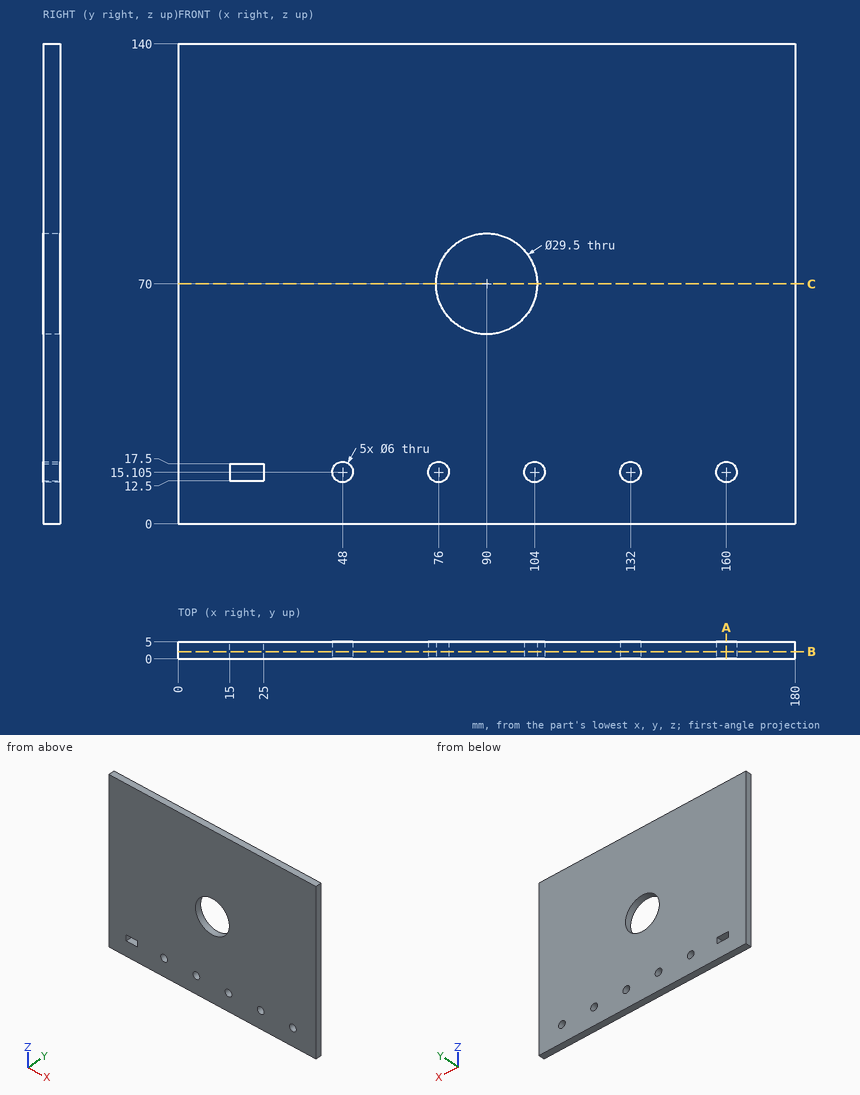
Study the drawing (mm; zero at the part's minimum x, y, z) and answer. Give positions to 0.01 mm unless a question says otherwise; leave off trailing zeros. Write each loop counter-clockwise with the first axis right and the second up, starting at its lowest first coordinate (ties: lowest second). Pieces come first, ordered by that corner, then holes. Notation, with made-up numbers: (31, 23.25) - (80, 23.25) arc R16 cw to (80, 39.25) - close; hole circle Ø9 at (46, -35.75). An arc over 180 degrees is marked (long way). Use CSV: the item, a comma, the result in double quotes. Start each with the question number.
(1) Find section C-C (z = 70). Give the vertices of the cut face in (x, y).
(2) Find section B-B (y = 2.1). Give the vertices of the cut face in (x, z) (3 decimals).
(3) Consider line 1 along X through (y, z) = (2.8, 70); line 2 along Z through (x, y) = (20, 3.55); line 3 along X through (y, z) = (0.8, 75). Determine where each line is inside the solid, lowest interval first.
(4) Find section A-A (x = 160). Give the vertices of the cut face in (y, z) (3 decimals), plus the area to 3 significant figures.
Findings below:
1,outline,"(0, 0) - (75.25, 0) - (75.25, 5) - (0, 5) - close; (104.75, 0) - (180, 0) - (180, 5) - (104.75, 5) - close"
2,outline,"(0, 0) - (180, 0) - (180, 140) - (0, 140) - close; hole (15, 12.5) - (25, 12.5) - (25, 17.5) - (15, 17.5) - close; hole circle Ø6 at (48, 15.105); hole circle Ø6 at (76, 15.105); hole circle Ø29.5 at (90, 70); hole circle Ø6 at (104, 15.105); hole circle Ø6 at (132, 15.105); hole circle Ø6 at (160, 15.105)"
3,line 1,"0 to 75.25, 104.75 to 180"
3,line 2,"0 to 12.5, 17.5 to 140"
3,line 3,"0 to 76.12, 103.88 to 180"
4,outline,"(0, 0) - (5, 0) - (5, 12.105) - (0, 12.105) - close; (0, 18.105) - (5, 18.105) - (5, 140) - (0, 140) - close"
4,area,"670 mm2"
